Source: CAD feature listing. Evaluate the final solid. Frame: model axes, mm. A direction names the side the tool comes from. Round coordinates to 2 decimals unless told otherwise and drop trailing zeros. Loops run counter-clockwise (first coordinate to the right, second up) from the corner with the lowest first, then second, coordinate; pieces in that order, holes last. Notation, with made-up numbers: (-4, -29.5) -> (22, -29.5) arc R27 ccw to (22, -5.5) -> close; hole circle Ø5 at (50, 84). An arc over 180 degrees is marked (long way). Put each result on its own line as item: value. Start each with the question number.
1. Draft query along Z for faces 1 (the flat face through (2, 0, 27.5)), 2 (the flat face through (35, 0, 28)), 3 (the flat face through (0, 0, 30)). Return one class per face: pulls with the +Z half, pulls with the -Z half, needs draft (parallel to the pull), parting line crosses it, or undercut.
2. Contact query for a flat-ended pin moving along its axis: pin 1 (2 mm diameter, centred on y = 12, z = 7.5, fed in from +X). Output: stop coordinate, or through.
3. Cut plane A-A (x = -23). Return the cut outline in (y, z).
4. Cut plane B-B (y = 1). Return the cut outline in (x, z), then the cut area to 3 significant figures.
5. Set-up query: faces 4 (the flat face through (-35, 0, 16)), 5 (the flat face through (2, 0, 2.5)). Return all of +Z, -Z, +X, -X, +Y, -Y with unobstructed straight access to the full face (end or side cutting, diameter ignored); none if empty.
6. Material intervals for L1, parallel to Y at x = -23, z = 13.5; L2, parallel to Z at x = -26.5, y = 12.5; L3, parallel to X at y = -8, z = 17, sorted ascending.
7. Cut plane C-C (z = 23.75). Return the cut outline in (x, y).
```python
from build123d import *

# Parameters (mm, degrees)
SKETCH_W     = 70
SKETCH_H     = 50
PAD_DEPTH    = 30
SKETCH001_W  = 45
SKETCH001_H  = 25
POCKET_DEPTH = 67
FILLET_R     = 1.5
FILLET001_R  = 1.5
FILLET002_R  = 1.5
FILLET003_R  = 1.5


with BuildPart() as part:
    # Sketch → Pad (new body)
    with BuildSketch(Plane.XY):
        Rectangle(SKETCH_W, SKETCH_H)
    extrude(amount=PAD_DEPTH)

    # Sketch001 (on Face2 of Pad) → Pocket (cut)
    with BuildSketch(Plane.YZ.offset(35)):
        with Locations((0, 15)):
            Rectangle(SKETCH001_W, SKETCH001_H)
    extrude(amount=-POCKET_DEPTH, mode=Mode.SUBTRACT)

    # Fillet
    fillet_edges = [part.edges().sort_by_distance(p)[0] for p in [
        (-35, 0, 0),
    ]]
    fillet(fillet_edges, radius=FILLET_R)

    # Fillet001
    fillet001_edges = [part.edges().sort_by_distance(p)[0] for p in [
        (35, 0, 0),
    ]]
    fillet(fillet001_edges, radius=FILLET001_R)

    # Fillet002
    fillet002_edges = [part.edges().sort_by_distance(p)[0] for p in [
        (0, -25, 0),
    ]]
    fillet(fillet002_edges, radius=FILLET002_R)

    # Fillet003
    fillet003_edges = [part.edges().sort_by_distance(p)[0] for p in [
        (0, 25, 0),
    ]]
    fillet(fillet003_edges, radius=FILLET003_R)


solid = part.part
```
Solution:
1. face 1: undercut
1. face 2: needs draft
1. face 3: pulls with the +Z half
2. pin 1: stops at x = -32
3. outline: (-25, 1.5) arc R1.5 ccw to (-23.5, 0) -> (23.5, 0) arc R1.5 ccw to (25, 1.5) -> (25, 30) -> (-25, 30) -> close; hole (-22.5, 2.5) -> (22.5, 2.5) -> (22.5, 27.5) -> (-22.5, 27.5) -> close
4. outline: (-35, 1.5) arc R1.5 ccw to (-33.5, 0) -> (33.5, 0) arc R1.5 ccw to (35, 1.5) -> (35, 2.5) -> (-32, 2.5) -> (-32, 27.5) -> (35, 27.5) -> (35, 30) -> (-35, 30) -> close
4. area: 424 mm^2
5. face 4: +Z, -Z, -X, +Y, -Y
5. face 5: +X
6. L1: y = -25 to -22.5, 22.5 to 25
6. L2: z = 0 to 2.5, 27.5 to 30
6. L3: x = -35 to -32
7. outline: (-35, -23.5) arc R1.5 ccw to (-33.5, -25) -> (33.5, -25) arc R1.5 ccw to (35, -23.5) -> (35, -22.5) -> (-32, -22.5) -> (-32, 22.5) -> (35, 22.5) -> (35, 23.5) arc R1.5 ccw to (33.5, 25) -> (-33.5, 25) arc R1.5 ccw to (-35, 23.5) -> close
